```python
from build123d import *

# Parameters (mm, degrees)
F0_W          = 9.525
F0_H          = 88.9
F1_DEPTH      = 88.9
F2_R          = 25.4
F3_DEPTH      = 69.85
F3_DEPTH_BACK = 30.734
F4_DEPTH      = 12.192
F5_R          = 12.7
F6_DEPTH      = 42.1005
F7_R          = 12.7
F8_DEPTH      = 35.6218531678
F9_R          = 25.4
F10_DEPTH     = 40.9996094773
F11_R         = 12.7
F12_DEPTH     = 47.4110707312
F13_R         = 12.7
F14_DEPTH     = 40.5094634056
F16_DEPTH     = 263.7934967819
F17_R         = 25.4
F18_DEPTH     = 50.8
F19_DEPTH     = 2.54


with BuildPart() as f1:
    # F0 (on Right) → F1 (new body)
    with BuildSketch(Plane.YZ):
        with Locations((46.1899, 0)):
            Rectangle(F0_W, F0_H)
    extrude(amount=F1_DEPTH)



with BuildPart() as f1b:
    # F0 (on Right) → F1, piece 2 (new body)
    with BuildSketch(Plane.YZ):
        with Locations((73.9394, 0)):
            Rectangle(F0_W, F0_H)
    extrude(amount=F1_DEPTH)


with BuildPart() as f1c:
    # F0 (on Right) → F1, piece 3 (new body)
    with BuildSketch(Plane.YZ):
        with Locations((125.5649, 0)):
            Rectangle(F0_W, F0_H)
    extrude(amount=F1_DEPTH)


with BuildPart() as f1d:
    # F0 (on Right) → F1, piece 4 (new body)
    with BuildSketch(Plane.YZ):
        with Locations((170.7117531678, 0)):
            Rectangle(F0_W, F0_H)
    extrude(amount=F1_DEPTH)


with BuildPart() as f1e:
    # F0 (on Right) → F1, piece 5 (new body)
    with BuildSketch(Plane.YZ):
        with Locations((221.2363626451, 0)):
            Rectangle(F0_W, F0_H)
    extrude(amount=F1_DEPTH)


with BuildPart() as f1f:
    # F0 (on Right) → F1, piece 6 (new body)
    with BuildSketch(Plane.YZ):
        with Locations((278.1724333763, 0)):
            Rectangle(F0_W, F0_H)
    extrude(amount=F1_DEPTH)


with BuildPart() as f1g:
    # F0 (on Right) → F1, piece 7 (new body)
    with BuildSketch(Plane.YZ):
        with Locations((328.2068967819, 0)):
            Rectangle(F0_W, F0_H)
    extrude(amount=F1_DEPTH)


with BuildPart() as f1_1:
    add(f1.part)

    add(f1b.part)  # F3 merges F1b
    # F2 (on face) → F3 (join, two sides)
    with BuildSketch(Plane.XZ.offset(-41.4274)) as f3_sk:
        with Locations((44.45, 0)):
            Circle(F2_R)
    extrude(amount=F3_DEPTH)
    extrude(f3_sk.sketch, amount=-F3_DEPTH_BACK)

    # F2 (on face) → F4 (cut)
    with BuildSketch(Plane.XZ.offset(-41.4274)):
        with BuildLine():
            ThreePointArc((44.45, 44.45), (75.8808964237, 31.4308964237), (88.9, 0))
            Line((88.9, 0), (88.9, 44.45))
            Line((88.9, 44.45), (44.45, 44.45))
        make_face()
        with BuildLine():
            ThreePointArc((0, -1.192e-07), (13.0191035341, 31.4308963816), (44.45, 44.45))
            Line((44.45, 44.45), (0, 44.45))
            Line((0, 44.45), (0, -1.192e-07))
        make_face()
        with BuildLine():
            Line((0, -44.45), (44.45, -44.45))
            ThreePointArc((44.45, -44.45), (13.0191036184, -31.4308964659), (0, -1.192e-07))
            Line((0, -1.192e-07), (0, -44.45))
        make_face()
        with BuildLine():
            Line((88.9, -44.45), (88.9, 0))
            ThreePointArc((88.9, 0), (75.8808964237, -31.4308964237), (44.45, -44.45))
            Line((44.45, -44.45), (88.9, -44.45))
        make_face()
    extrude(amount=-F4_DEPTH, mode=Mode.SUBTRACT)


    add(f1c.part)  # F6 merges F1c
    # F5 (on face) → F6 (join, through all)
    with BuildSketch(Plane.XZ.offset(-120.8024)):
        with Locations((44.45, 25.4)):
            Circle(F5_R)
    extrude(amount=F6_DEPTH)


    add(f1d.part)  # F8 merges F1d
    # F7 (on face) → F8 (join, through all)
    with BuildSketch(Plane(origin=(0, 130.3274, 0), x_dir=(-1, 0, 0), z_dir=(0, 1, 0))):
        with Locations((-44.45, -25.4)):
            Circle(F7_R)
    extrude(amount=F8_DEPTH)


    add(f1e.part)  # F10 merges F1e
    # F9 (on face) → F10 (join, through all)
    with BuildSketch(Plane(origin=(0, 175.4742531678, 0), x_dir=(-1, 0, 0), z_dir=(0, 1, 0))):
        with Locations((-44.45, 0)):
            Circle(F9_R)
    extrude(amount=F10_DEPTH)


    add(f1f.part)  # F12 merges F1f
    # F11 (on face) → F12 (join, through all)
    with BuildSketch(Plane(origin=(0, 225.9988626451, 0), x_dir=(-1, 0, 0), z_dir=(0, 1, 0))):
        with Locations((-44.45, 25.4)):
            Circle(F11_R)
    extrude(amount=F12_DEPTH)


    add(f1g.part)  # F14 merges F1g
    # F13 (on face) → F14 (join, through all)
    with BuildSketch(Plane(origin=(0, 282.9349333763, 0), x_dir=(-1, 0, 0), z_dir=(0, 1, 0))):
        with Locations((-44.45, -25.4)):
            Circle(F13_R)
    extrude(amount=F14_DEPTH)

    # F15 (on face) → F16 (cut, through all)
    with BuildSketch(Plane.XZ.offset(-69.1769)):
        with BuildLine():
            ThreePointArc((0, 3.5263449072), (12.9203503952, 31.5296496048), (40.9236550928, 44.45))
            Line((40.9236550928, 44.45), (0, 44.45))
            Line((0, 44.45), (0, 3.5263449072))
        make_face()
        with BuildLine():
            Line((0, -44.45), (40.9236550928, -44.45))
            ThreePointArc((40.9236550928, -44.45), (12.9203503952, -31.5296496048), (0, -3.5263449072))
            Line((0, -3.5263449072), (0, -44.45))
        make_face()
        with BuildLine():
            Line((88.9, -44.45), (88.9, -3.5263449072))
            ThreePointArc((88.9, -3.5263449072), (75.9796496048, -31.5296496048), (47.9763449072, -44.45))
            Line((47.9763449072, -44.45), (88.9, -44.45))
        make_face()
        with BuildLine():
            ThreePointArc((47.9763449072, 44.45), (75.9796496048, 31.5296496048), (88.9, 3.5263449072))
            Line((88.9, 3.5263449072), (88.9, 44.45))
            Line((88.9, 44.45), (47.9763449072, 44.45))
        make_face()
    extrude(amount=-F16_DEPTH, mode=Mode.SUBTRACT)

    # F17 (on face) → F18 (join)
    with BuildSketch(Plane(origin=(0, 332.9693967819, 0), x_dir=(-1, 0, 0), z_dir=(0, 1, 0))):
        with Locations((-44.45, 0)):
            Circle(F17_R)
    extrude(amount=F18_DEPTH)

    # F19 (cut): a face of the model
    f19_faces = [f1_1.faces().sort_by_distance(p)[0] for p in [
        (44.45, 78.7019, -2.2434372105),
    ]]
    extrude(f19_faces, amount=-F19_DEPTH, mode=Mode.SUBTRACT)


solid = f1_1.part
```
CAD build for the part. Positions are in the model's coordinates, mm. A direction names the side the tool comes from. Round coordinates to 2 decimals unless told otherwise and drop trailing zeros. Order: outer loops, then holes, each group sorted by start corner. A loop starts at its lowest first (then second) coordinate and runs counter-clockwise, first axis right, second up.
Item 1: Tool access for faces 1 (the face through (64.607, 358.014, -15.456)), 2 (the face through (76.29, 170.645, -31.216)), 3 (the face through (56.171, 6.991, -22.534)), 4 (the face through (53.81, 249.373, 33.983)): list every direction of +Z, -Z, +X, -X, +Y, -Y with a clear straight run to the whole face (end or side of a thin tool).
Item 2: Pin check, flat tips, straight feed: pin 1 (10 mm diameter, centred on x = 26, y = 327.5, fed in from +Z); pin 2 (4 mm diameter, centred on x = 75.5, z = -10.5, fed in from -Y); pin 3 (6 mm diameter, centred on x = 27, y = 44.5, fed in from +Z). Stop position of each tip, or through.
Item 3: Saw through at C-C on y = 46.5. Write the cut outline in (x, z), then the cut area to 3 significant figures.
Item 4: Probe line 1 along Y through (x, z) = (33.5, 14.5); line 2 along Y through (x, z) = (43.5, 13); line 3 along Y through (x, z) = (45.5, -17). List the from-to ranges inside material, lowest first.
Item 5: Mould opens along Y. For faces 5 (the face through (45, 383.769, 0)), 6 (the face through (64, 175.474, 19)), 7 (the face through (12.61, 170.645, 31.216)) say: pulls with the +Y half, pulls with the -Y half, needs draft (parallel to the pull), parting line crosses it, or undercut.
Item 6: Saw through at B-B on y = -1. Write the cut outline in (x, z).
Item 7: Saw through at A-A on x = 12. Write the cut outline in (y, z), then the cut area to 3 significant figures.
Reported:
1. face 1: +Y
1. face 2: -Z, +X, +Y, -Y
1. face 3: -Y
1. face 4: none
2. pin 1: stops at z = 42.51
2. pin 2: stops at y = 41.43
2. pin 3: stops at z = 42.04
3. outline: circle Ø88.9 at (44.45, 0)
3. area: 6,210 mm2
4. line 1: y = -28.42 to 76.16, 120.8 to 130.33, 165.95 to 226, 273.41 to 282.93, 323.44 to 383.77
4. line 2: y = -28.42 to 130.33, 165.95 to 282.93, 323.44 to 383.77
4. line 3: y = -28.42 to 76.16, 120.8 to 226, 273.41 to 383.77
5. face 5: pulls with the +Y half
5. face 6: undercut
5. face 7: needs draft
6. outline: circle Ø50.8 at (44.45, 0)
7. outline: (41.43, -30.38) - (50.95, -30.38) - (50.95, 30.38) - (41.43, 30.38) - close; (69.18, -30.58) - (76.16, -30.58) - (76.16, 30.58) - (69.18, 30.58) - close; (120.8, -30.58) - (130.33, -30.58) - (130.33, 30.58) - (120.8, 30.58) - close; (165.95, -30.58) - (175.47, -30.58) - (175.47, 30.58) - (165.95, 30.58) - close; (216.47, -30.58) - (226, -30.58) - (226, 30.58) - (216.47, 30.58) - close; (273.41, -30.58) - (282.93, -30.58) - (282.93, 30.58) - (273.41, 30.58) - close; (323.44, -30.58) - (332.97, -30.58) - (332.97, 30.58) - (323.44, 30.58) - close
7. area: 3,920 mm2
